The model under review builds one solid part; all positions refer to its coordinate system, in mm. A direction names the side the tool comes from. Coordinates: 2 decimals unless noted, no trailing zeros. Order: outer loops, then holes, each group sorted by start corner. A loop starts at its lowest first (then second) coordinate and runs counter-clockwise, first axis right, second up. Notation, with made-up numbers: (10.5, 24.5) -> (20.5, 24.5) arc R17 ccw to (20.5, 47.5) -> close; hole circle Ø5 at (11, -26). An arc over 180 degrees is marked (long way). Put each result on its own line as item: value.
from build123d import *
from OCP.BRepFilletAPI import BRepFilletAPI_MakeChamfer

# Parameters (mm, degrees)
SKETCH2_W                     = 14
SKETCH2_H                     = 19
BOSS_EXTRUDE1_DEPTH           = 1.5
SKETCH3_R                     = 1.5
CUT_EXTRUDE1_DEPTH            = 12.895377253
SKETCH4_W                     = 13
SKETCH4_H                     = 2.5
BOSS_EXTRUDE2_DEPTH           = 2.5
SKETCH5_W                     = 0.5
SKETCH5_H                     = 0.5
BOSS_EXTRUDE3_DEPTH           = 5.5
CHAMFER1_SIZE                 = 0.3
CHAMFER1_SIZE2                = 0.10919107
SKETCH6_W                     = 12.5
SKETCH6_H                     = 5.5
SKETCH6_W_2                   = 4.5
SKETCH6_H_2                   = 1.5
SKETCH6_W_3                   = 2.5
SKETCH6_H_3                   = 1
KOPONENTTIEN_TILAVARAUS_DEPTH = 1


with BuildPart() as part:
    # Sketch2 → Boss-Extrude1 (new body)
    with BuildSketch(Plane.XY):
        Rectangle(SKETCH2_W, SKETCH2_H)
    extrude(amount=BOSS_EXTRUDE1_DEPTH)

    # Sketch3 → Cut-Extrude1 (cut, through all)
    with BuildSketch(Plane.XY.offset(1.5)):
        with Locations((-4.25, 6)):
            Circle(SKETCH3_R)
        with Locations(Location((4.25, 6, 0), (0, 0, 180))):
            Circle(SKETCH3_R)
    extrude(amount=-CUT_EXTRUDE1_DEPTH, mode=Mode.SUBTRACT)

    # Sketch4 → Boss-Extrude2 (add)
    with BuildSketch(Plane.XY.offset(1.5)):
        with Locations((0, -7.75)):
            Rectangle(SKETCH4_W, SKETCH4_H)
    extrude(amount=BOSS_EXTRUDE2_DEPTH)

    # Sketch5 → Boss-Extrude3 (add)
    with BuildSketch(Plane.XY.offset(4)):
        with Locations((-5.08, -7.75)):
            Rectangle(SKETCH5_W, SKETCH5_H)
        with Locations((-2.54, -7.75)):
            Rectangle(SKETCH5_W, SKETCH5_H)
        with Locations((0, -7.75)):
            Rectangle(SKETCH5_W, SKETCH5_H)
        with Locations((2.54, -7.75)):
            Rectangle(SKETCH5_W, SKETCH5_H)
        with Locations((5.08, -7.75)):
            Rectangle(SKETCH5_W, SKETCH5_H)
    extrude(amount=BOSS_EXTRUDE3_DEPTH)

    # Chamfer1: one chamfer whose edges measure the first distance from different faces: ONE call of the kernel's chamfer builder (chamfer() names one face for all edges)
    chamfer1_edges_1 = [part.edges().sort_by_distance(p)[0] for p in [
        (-4.83, -7.75, 9.5),
    ]]
    chamfer1_side_1 = [part.faces().sort_by_distance(p)[0] for p in [
        (-4.83, -7.75, 6.75),
    ]]
    chamfer1_edges_2 = [part.edges().sort_by_distance(p)[0] for p in [
        (-5.08, -7.5, 9.5),
    ]]
    chamfer1_side_2 = [part.faces().sort_by_distance(p)[0] for p in [
        (-5.08, -7.5, 6.75),
    ]]
    chamfer1_edges_3 = [part.edges().sort_by_distance(p)[0] for p in [
        (-5.33, -7.75, 9.5),
    ]]
    chamfer1_side_3 = [part.faces().sort_by_distance(p)[0] for p in [
        (-5.33, -7.75, 6.75),
    ]]
    chamfer1_edges_4 = [part.edges().sort_by_distance(p)[0] for p in [
        (-5.08, -8, 9.5),
    ]]
    chamfer1_side_4 = [part.faces().sort_by_distance(p)[0] for p in [
        (-5.08, -8, 6.75),
    ]]
    chamfer1_edges_5 = [part.edges().sort_by_distance(p)[0] for p in [
        (-2.29, -7.75, 9.5),
    ]]
    chamfer1_side_5 = [part.faces().sort_by_distance(p)[0] for p in [
        (-2.29, -7.75, 6.75),
    ]]
    chamfer1_edges_6 = [part.edges().sort_by_distance(p)[0] for p in [
        (-2.54, -7.5, 9.5),
    ]]
    chamfer1_side_6 = [part.faces().sort_by_distance(p)[0] for p in [
        (-2.54, -7.5, 6.75),
    ]]
    chamfer1_edges_7 = [part.edges().sort_by_distance(p)[0] for p in [
        (-2.79, -7.75, 9.5),
    ]]
    chamfer1_side_7 = [part.faces().sort_by_distance(p)[0] for p in [
        (-2.79, -7.75, 6.75),
    ]]
    chamfer1_edges_8 = [part.edges().sort_by_distance(p)[0] for p in [
        (-2.54, -8, 9.5),
    ]]
    chamfer1_side_8 = [part.faces().sort_by_distance(p)[0] for p in [
        (-2.54, -8, 6.75),
    ]]
    chamfer1_edges_9 = [part.edges().sort_by_distance(p)[0] for p in [
        (0.25, -7.75, 9.5),
    ]]
    chamfer1_side_9 = [part.faces().sort_by_distance(p)[0] for p in [
        (0.25, -7.75, 6.75),
    ]]
    chamfer1_edges_10 = [part.edges().sort_by_distance(p)[0] for p in [
        (0, -7.5, 9.5),
    ]]
    chamfer1_side_10 = [part.faces().sort_by_distance(p)[0] for p in [
        (0, -7.5, 6.75),
    ]]
    chamfer1_edges_11 = [part.edges().sort_by_distance(p)[0] for p in [
        (-0.25, -7.75, 9.5),
    ]]
    chamfer1_side_11 = [part.faces().sort_by_distance(p)[0] for p in [
        (-0.25, -7.75, 6.75),
    ]]
    chamfer1_edges_12 = [part.edges().sort_by_distance(p)[0] for p in [
        (0, -8, 9.5),
    ]]
    chamfer1_side_12 = [part.faces().sort_by_distance(p)[0] for p in [
        (0, -8, 6.75),
    ]]
    chamfer1_edges_13 = [part.edges().sort_by_distance(p)[0] for p in [
        (2.79, -7.75, 9.5),
    ]]
    chamfer1_side_13 = [part.faces().sort_by_distance(p)[0] for p in [
        (2.79, -7.75, 6.75),
    ]]
    chamfer1_edges_14 = [part.edges().sort_by_distance(p)[0] for p in [
        (2.54, -7.5, 9.5),
    ]]
    chamfer1_side_14 = [part.faces().sort_by_distance(p)[0] for p in [
        (2.54, -7.5, 6.75),
    ]]
    chamfer1_edges_15 = [part.edges().sort_by_distance(p)[0] for p in [
        (2.29, -7.75, 9.5),
    ]]
    chamfer1_side_15 = [part.faces().sort_by_distance(p)[0] for p in [
        (2.29, -7.75, 6.75),
    ]]
    chamfer1_edges_16 = [part.edges().sort_by_distance(p)[0] for p in [
        (2.54, -8, 9.5),
    ]]
    chamfer1_side_16 = [part.faces().sort_by_distance(p)[0] for p in [
        (2.54, -8, 6.75),
    ]]
    chamfer1_edges_17 = [part.edges().sort_by_distance(p)[0] for p in [
        (5.33, -7.75, 9.5),
    ]]
    chamfer1_side_17 = [part.faces().sort_by_distance(p)[0] for p in [
        (5.33, -7.75, 6.75),
    ]]
    chamfer1_edges_18 = [part.edges().sort_by_distance(p)[0] for p in [
        (5.08, -7.5, 9.5),
    ]]
    chamfer1_side_18 = [part.faces().sort_by_distance(p)[0] for p in [
        (5.08, -7.5, 6.75),
    ]]
    chamfer1_edges_19 = [part.edges().sort_by_distance(p)[0] for p in [
        (4.83, -7.75, 9.5),
    ]]
    chamfer1_side_19 = [part.faces().sort_by_distance(p)[0] for p in [
        (4.83, -7.75, 6.75),
    ]]
    chamfer1_edges_20 = [part.edges().sort_by_distance(p)[0] for p in [
        (5.08, -8, 9.5),
    ]]
    chamfer1_side_20 = [part.faces().sort_by_distance(p)[0] for p in [
        (5.08, -8, 6.75),
    ]]
    chamfer1 = BRepFilletAPI_MakeChamfer(part.part.solid().wrapped)
    for e in chamfer1_edges_1:
        chamfer1.Add(CHAMFER1_SIZE, CHAMFER1_SIZE2, e.wrapped, chamfer1_side_1[0].wrapped)  # the first distance lies on this face
    for e in chamfer1_edges_2:
        chamfer1.Add(CHAMFER1_SIZE, CHAMFER1_SIZE2, e.wrapped, chamfer1_side_2[0].wrapped)  # the first distance lies on this face
    for e in chamfer1_edges_3:
        chamfer1.Add(CHAMFER1_SIZE, CHAMFER1_SIZE2, e.wrapped, chamfer1_side_3[0].wrapped)  # the first distance lies on this face
    for e in chamfer1_edges_4:
        chamfer1.Add(CHAMFER1_SIZE, CHAMFER1_SIZE2, e.wrapped, chamfer1_side_4[0].wrapped)  # the first distance lies on this face
    for e in chamfer1_edges_5:
        chamfer1.Add(CHAMFER1_SIZE, CHAMFER1_SIZE2, e.wrapped, chamfer1_side_5[0].wrapped)  # the first distance lies on this face
    for e in chamfer1_edges_6:
        chamfer1.Add(CHAMFER1_SIZE, CHAMFER1_SIZE2, e.wrapped, chamfer1_side_6[0].wrapped)  # the first distance lies on this face
    for e in chamfer1_edges_7:
        chamfer1.Add(CHAMFER1_SIZE, CHAMFER1_SIZE2, e.wrapped, chamfer1_side_7[0].wrapped)  # the first distance lies on this face
    for e in chamfer1_edges_8:
        chamfer1.Add(CHAMFER1_SIZE, CHAMFER1_SIZE2, e.wrapped, chamfer1_side_8[0].wrapped)  # the first distance lies on this face
    for e in chamfer1_edges_9:
        chamfer1.Add(CHAMFER1_SIZE, CHAMFER1_SIZE2, e.wrapped, chamfer1_side_9[0].wrapped)  # the first distance lies on this face
    for e in chamfer1_edges_10:
        chamfer1.Add(CHAMFER1_SIZE, CHAMFER1_SIZE2, e.wrapped, chamfer1_side_10[0].wrapped)  # the first distance lies on this face
    for e in chamfer1_edges_11:
        chamfer1.Add(CHAMFER1_SIZE, CHAMFER1_SIZE2, e.wrapped, chamfer1_side_11[0].wrapped)  # the first distance lies on this face
    for e in chamfer1_edges_12:
        chamfer1.Add(CHAMFER1_SIZE, CHAMFER1_SIZE2, e.wrapped, chamfer1_side_12[0].wrapped)  # the first distance lies on this face
    for e in chamfer1_edges_13:
        chamfer1.Add(CHAMFER1_SIZE, CHAMFER1_SIZE2, e.wrapped, chamfer1_side_13[0].wrapped)  # the first distance lies on this face
    for e in chamfer1_edges_14:
        chamfer1.Add(CHAMFER1_SIZE, CHAMFER1_SIZE2, e.wrapped, chamfer1_side_14[0].wrapped)  # the first distance lies on this face
    for e in chamfer1_edges_15:
        chamfer1.Add(CHAMFER1_SIZE, CHAMFER1_SIZE2, e.wrapped, chamfer1_side_15[0].wrapped)  # the first distance lies on this face
    for e in chamfer1_edges_16:
        chamfer1.Add(CHAMFER1_SIZE, CHAMFER1_SIZE2, e.wrapped, chamfer1_side_16[0].wrapped)  # the first distance lies on this face
    for e in chamfer1_edges_17:
        chamfer1.Add(CHAMFER1_SIZE, CHAMFER1_SIZE2, e.wrapped, chamfer1_side_17[0].wrapped)  # the first distance lies on this face
    for e in chamfer1_edges_18:
        chamfer1.Add(CHAMFER1_SIZE, CHAMFER1_SIZE2, e.wrapped, chamfer1_side_18[0].wrapped)  # the first distance lies on this face
    for e in chamfer1_edges_19:
        chamfer1.Add(CHAMFER1_SIZE, CHAMFER1_SIZE2, e.wrapped, chamfer1_side_19[0].wrapped)  # the first distance lies on this face
    for e in chamfer1_edges_20:
        chamfer1.Add(CHAMFER1_SIZE, CHAMFER1_SIZE2, e.wrapped, chamfer1_side_20[0].wrapped)  # the first distance lies on this face
    add(Compound.cast(chamfer1.Shape()), mode=Mode.REPLACE)

    # Sketch6 → Koponenttien tilavaraus (add)
    with BuildSketch(Plane(origin=(0, 0, 0), x_dir=(-1, 0, 0), z_dir=(0, 0, -1))):
        with Locations((0, -6.25)):
            Rectangle(SKETCH6_W, SKETCH6_H)
        with Locations((0, 1.75)):
            Rectangle(SKETCH6_W_2, SKETCH6_H_2)
        with Locations((0, 6)):
            Rectangle(SKETCH6_W_3, SKETCH6_H_3)
        with Locations((0, 4.5)):
            Rectangle(SKETCH6_W_3, SKETCH6_H_3)
    extrude(amount=KOPONENTTIEN_TILAVARAUS_DEPTH)


solid = part.part
Item 1: Consider section C-C on x = 4.25. Write out the cut boundary in (y, z), and give its area (4 significant figures).
Answers below:
outline: (-9.5, 0) -> (-9, 0) -> (-9, -1) -> (-3.5, -1) -> (-3.5, 0) -> (4.5, 0) -> (4.5, 1.5) -> (-6.5, 1.5) -> (-6.5, 4) -> (-9, 4) -> (-9, 1.5) -> (-9.5, 1.5) -> close; (7.5, 0) -> (9.5, 0) -> (9.5, 1.5) -> (7.5, 1.5) -> close
area: 35.75 mm^2
Item 2: Consider section B-B on y = 6. Write out the cut boundary in (x, z).
Answers below:
outline: (-7, 0) -> (-5.75, 0) -> (-5.75, 1.5) -> (-7, 1.5) -> close; (-2.75, 0) -> (-1.25, 0) -> (-1.25, -1) -> (1.25, -1) -> (1.25, 0) -> (2.75, 0) -> (2.75, 1.5) -> (-2.75, 1.5) -> close; (5.75, 0) -> (7, 0) -> (7, 1.5) -> (5.75, 1.5) -> close
Item 3: Consider section A-A on z = 4.5. Write out the cut boundary in (x, y).
Answers below:
outline: (-5.33, -8) -> (-4.83, -8) -> (-4.83, -7.5) -> (-5.33, -7.5) -> close; (-2.79, -8) -> (-2.29, -8) -> (-2.29, -7.5) -> (-2.79, -7.5) -> close; (-0.25, -8) -> (0.25, -8) -> (0.25, -7.5) -> (-0.25, -7.5) -> close; (2.29, -8) -> (2.79, -8) -> (2.79, -7.5) -> (2.29, -7.5) -> close; (4.83, -8) -> (5.33, -8) -> (5.33, -7.5) -> (4.83, -7.5) -> close
Item 4: For line 1 (Y direction, x = 4.25, z = 1.25); line 2 (Z direction, x = 5.5, y = -6.75); line 3 (Z direction, x = 5.25, y = 0.25), list the stretches that pass through material, from the lowest coordinate up. Write a range as from..to.
Answers below:
line 1: -9.5..4.5, 7.5..9.5
line 2: -1..4
line 3: 0..1.5
Item 5: Mouldability with a two-part tool opening along Y and no side actions: class faces 1 (the flat face through (-6.25, -6.3, -0.5)), 2 (the flat face through (0, 6.5, -0.5)), 3 (the flat face through (0, 2.5, -0.5)), 4 (the cylindrical face through (2.82, 5.55, 0.76)) as +Y half, -Y half, draft (parallel to the pull), parting line (faces both ways), or undercut.
Answers below:
face 1: draft
face 2: +Y half
face 3: undercut
face 4: undercut
Item 6: Consider section D-D on x = 1.5. Write out the cut boundary in (y, z), and give its area (4 significant figures).
Answers below:
outline: (-9.5, 0) -> (-9, 0) -> (-9, -1) -> (-3.5, -1) -> (-3.5, 0) -> (1, 0) -> (1, -1) -> (2.5, -1) -> (2.5, 0) -> (9.5, 0) -> (9.5, 1.5) -> (-6.5, 1.5) -> (-6.5, 4) -> (-9, 4) -> (-9, 1.5) -> (-9.5, 1.5) -> close
area: 41.75 mm^2
Item 7: For faces 5 (the flat face through (6.25, -6.3, -0.5)), 6 (the flat face through (0, -9, 3)), 7 (the flat face through (-2.25, 1.7, -0.5)), 8 (the flat face through (1.25, 4.5, -0.5)), list the 3-axis set-ups (+Z, -Z, +X, -X, +Y, -Y) from which the entire face can be reached by the end or side of a thin tool; tool diameter is ignored.
Answers below:
face 5: -Z, +X, +Y, -Y
face 6: +Z, +X, -X, -Y
face 7: -Z, -X, +Y
face 8: -Z, +X, +Y
Item 8: For pin 1 Ø2 at (x, y) = (3.5, 3) entering from +Z; pin 2 Ø0.6 at (x, z) = (0, 7) entering from -Y; pin 3 Ø0.5 at (y, z) = (4.5, -0.5) entering from -X, all flat-tipped, find the tip position at first contact; note any pin that passes through.
Answers below:
pin 1: z = 1.5
pin 2: y = -8
pin 3: x = -1.25
